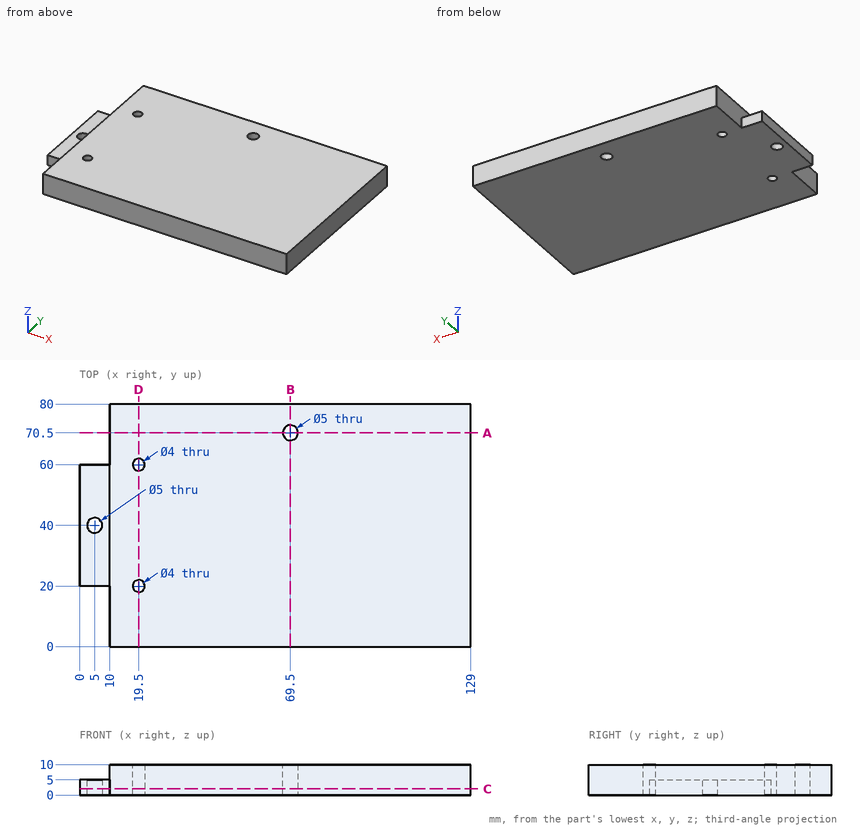
Answer from the drawing. Dimensions are ordinates in mm from the lowest x, y and z of the part. Round coordinates to 2 decimals unless told otherwise and drop trailing zeros. Order: outer loops, then holes, each group sorted by start corner. A loop starts at its lowest first (then second) coordinate and runs counter-clockwise, first axis right, second up. Notation, with made-up numbers: (-39, 60.25) - (16, 60.25) arc R30 ccw to (16, 82.25) - close; hole circle Ø1 at (-28.5, -23.5). An arc over 180 degrees is marked (long way). Put each result on its own line as item: value. Start each with the question number.
(1) Find section A-A (y = 70.5). Give the vertices of the cut face in (x, z), plus the area to 3 significant figures.
(2) Straight lines are drawn through the part: probe 1 along Y at (x, z) = (19.5, 2.5); probe 2 along Y at (x, z) = (69.5, 3); probe 3 along X at (y, z) = (29, 8.5). For each, find the intervals that lie inside material, in ascending order. Write a range as from..to.
(3) Find section D-D (x = 19.5). Give the vertices of the cut face in (y, z).
(4) Find section B-B (x = 69.5). Give the vertices of the cut face in (y, z).
(5) Find section C-C (z = 2). Give the vertices of the cut face in (x, y).
(6) Given P1, Ø6, axis at x = 32, z = 2, coming from the -Y side; P2, Ø5.5, axis at x = 3, z = 2, coming from the -Y side; P3, Ø3, axis at y = 46.5, z = 7.5, coming from the -X side; P4, Ø5, axis at x = 6.5, y = 34, coming from the +Z side, each flat-ended and moving along its own axis, determine where each tip first touches the part or whether it passes through.
Reply:
1. outline: (10, 0) - (67, 0) - (67, 10) - (10, 10) - close; (72, 0) - (129, 0) - (129, 10) - (72, 10) - close
1. area: 1,140 mm^2
2. probe 1: 0..18, 22..58, 62..80
2. probe 2: 0..68, 73..80
2. probe 3: 10..129
3. outline: (0, 0) - (18, 0) - (18, 10) - (0, 10) - close; (22, 0) - (58, 0) - (58, 10) - (22, 10) - close; (62, 0) - (80, 0) - (80, 10) - (62, 10) - close
4. outline: (0, 0) - (68, 0) - (68, 10) - (0, 10) - close; (73, 0) - (80, 0) - (80, 10) - (73, 10) - close
5. outline: (0, 20) - (10, 20) - (10, 0) - (129, 0) - (129, 80) - (10, 80) - (10, 60) - (0, 60) - close; hole circle Ø5 at (5, 40); hole circle Ø4 at (19.5, 20); hole circle Ø4 at (19.5, 60); hole circle Ø5 at (69.5, 70.5)
6. P1: y = 0
6. P2: y = 20
6. P3: x = 10
6. P4: z = 5
